Source: three-view drawing plus pictorial views. Frame: mm from the lowest corner of the part. Give positions to 0.01 mm unless a question says otherwise; leave off trailing zeros. Order: outer loops, then holes, each group sorted by start corner. A loop starts at its lowest first (then second) coordinate and runs counter-clockwise, first axis right, second up. Notation, with made-up numbers: (35, 20) -> (87, 20) arc R17 ccw to (87, 24) -> close; hole circle Ø9 at (-26.75, 72). An arc over 180 degrees is marked (long way). Answer in a Markdown table with one row per item.
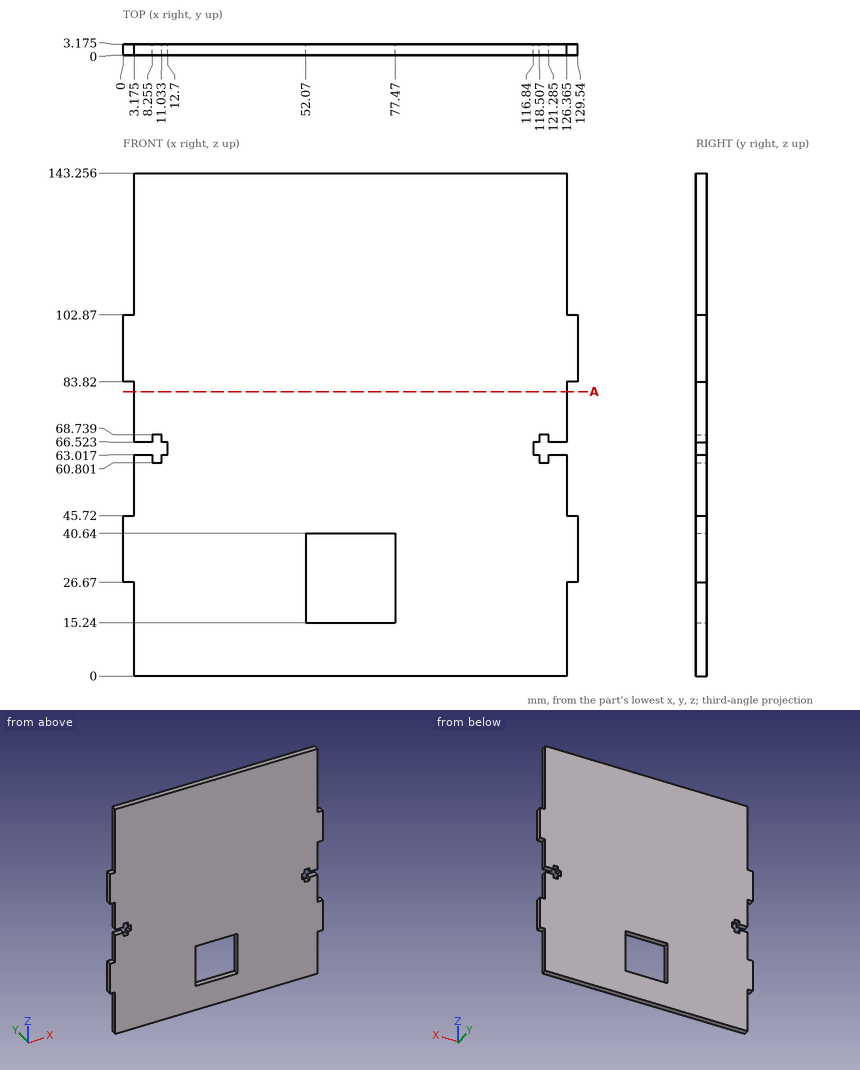
(1) Section query A-A (z = 81). Return the cut outline in (x, y) (1 decimal).
A:
| item | result |
|---|---|
| outline | (3.2, 0) -> (126.4, 0) -> (126.4, 3.2) -> (3.2, 3.2) -> close |
(2) First-contact query: pin 1 Ø1 at (x, y) = (1.5, 1) entering from +Z; pin 2 Ø1 at (y, z) = (2, 78) entering from +X (3 decimals); pin 3 Ø1.1 at (y, z) = (2, 61.5) entering from -X (3 decimals). Flat tips, straight axial feed; report the tip coordinate or a pass-through.
A:
| item | result |
|---|---|
| pin 1 | stops at z = 102.87 |
| pin 2 | stops at x = 126.365 |
| pin 3 | stops at x = 3.175 |
(3) Ray query, probe 1 along X at (y, z) = (1.45, 61) (1 decimal); probe 2 along Z at (x, y) = (73, 2.65); probe 3 along X at (y, z) = (0.95, 56.5) (1 decimal). Return the intervals inside material, ascending.
A:
| item | result |
|---|---|
| probe 1 | x = 3.2 to 8.3, 11 to 118.5, 121.3 to 126.4 |
| probe 2 | z = 0 to 15.24, 40.64 to 143.26 |
| probe 3 | x = 3.2 to 126.4 |
